Build history of the part. All positions in model axes, mm. Face numbers are marked on the shaded views. A direction names the side the tool comes from. Round coordinates to 2 decimals unless told otherwise and drop trailing zeros. Order: outer loops, then holes, each group sorted by start corner. A loop starts at its lowest first (then second) coordinate and runs counter-clockwise, first axis right, second up. Notation, with made-up numbers: M -36.75,52.5 L -17.75,52.5 A9 ccw -17.75,56.5 Z; hole C 35,-35.5 d2. An arc over 180 degrees is marked long. Use CSV: the item, a comma, the result in double quotes.
from build123d import *

# Parameters (mm, degrees)
EXTRUDE_1_DEPTH     = 10
EXTRUDE_2_DEPTH     = 10
FILLET_1_R          = 5
SKETCH_3_R          = 2.5
CUT_EXTRUDE_1_DEPTH = 10
SKETCH_4_R          = 2
CUT_EXTRUDE_2_DEPTH = 10
SKETCH_5_R          = 1.5
CUT_EXTRUDE_3_DEPTH = 10
SKETCH_6_R          = 10
CUT_EXTRUDE_4_DEPTH = 5


with BuildPart() as part:
    # 草图1 → 凸台-拉伸1 (new body)
    with BuildSketch(Plane(origin=(0, 0, 0), x_dir=(0, 0, -1), z_dir=(1, 0, 0))):
        with BuildLine():
            ThreePointArc((-7.942884534, 22.647529341), (-9.184402377, 22.17310878), (-10.397754058, 21.630689091))
            ThreePointArc((-10.397754058, 21.630689091), (-12.397305949, 24.184674774), (-15.156649968, 25.889688329))
            ThreePointArc((-15.156649968, 25.889688329), (-15.674956941, 25.579204931), (-16.186906117, 25.258346549))
            ThreePointArc((-16.186906117, 25.258346549), (-15.920443886, 22.02569307), (-14.552603542, 19.084594053))
            ThreePointArc((-14.552603542, 19.084594053), (-15.58675316, 18.249743174), (-16.573102281, 17.358925105))
            ThreePointArc((-16.573102281, 17.358925105), (-19.264014116, 19.170014316), (-22.41518439, 19.938894372))
            ThreePointArc((-22.41518439, 19.938894372), (-22.812178968, 19.48344145), (-23.199920874, 19.020085999))
            ThreePointArc((-23.199920874, 19.020085999), (-21.947555371, 16.027991201), (-19.737812321, 13.653525728))
            ThreePointArc((-19.737812321, 13.653525728), (-20.463363944, 12.539965553), (-21.126159781, 11.387948582))
            ThreePointArc((-21.126159781, 11.387948582), (-24.245026361, 12.278859291), (-27.479564388, 12.036342512))
            ThreePointArc((-27.479564388, 12.036342512), (-27.716385975, 11.480502971), (-27.941965733, 10.920006912))
            ThreePointArc((-27.941965733, 10.920006912), (-25.82628722, 8.46135788), (-22.990946508, 6.885955175))
            ThreePointArc((-22.990946508, 6.885955175), (-23.33687809, 5.602688733), (-23.611241567, 4.302240308))
            ThreePointArc((-23.611241567, 4.302240308), (-26.852766501, 4.185763967), (-29.854053162, 2.955589584))
            ThreePointArc((-29.854053162, 2.955589584), (-29.907520012, 2.353772872), (-29.948856303, 1.751001464))
            ThreePointArc((-29.948856303, 1.751001464), (-27.176962132, 0.066467896), (-23.993566664, -0.555660648))
            ThreePointArc((-23.993566664, -0.555660648), (-23.92601601, -1.883018297), (-23.785090519, -3.204601222))
            ThreePointArc((-23.785090519, -3.204601222), (-26.831970761, -4.317063099), (-29.306219208, -6.414477044))
            ThreePointArc((-29.306219208, -6.414477044), (-29.171097612, -7.003360916), (-29.024144152, -7.589404208))
            ThreePointArc((-29.024144152, -7.589404208), (-25.867366639, -8.334928429), (-22.647529341, -7.942884534))
            ThreePointArc((-22.647529341, -7.942884534), (-22.17310878, -9.184402377), (-21.630689091, -10.397754058))
            ThreePointArc((-21.630689091, -10.397754058), (-24.184674774, -12.397305949), (-25.889688329, -15.156649968))
            ThreePointArc((-25.889688329, -15.156649968), (-25.579204931, -15.674956941), (-25.258346549, -16.186906117))
            ThreePointArc((-25.258346549, -16.186906117), (-22.02569307, -15.920443886), (-19.084594053, -14.552603542))
            ThreePointArc((-19.084594053, -14.552603542), (-18.249743174, -15.58675316), (-17.358925105, -16.573102281))
            ThreePointArc((-17.358925105, -16.573102281), (-19.170014316, -19.264014116), (-19.938894372, -22.41518439))
            ThreePointArc((-19.938894372, -22.41518439), (-19.48344145, -22.812178968), (-19.020085999, -23.199920874))
            ThreePointArc((-19.020085999, -23.199920874), (-16.027991201, -21.947555371), (-13.653525728, -19.737812321))
            ThreePointArc((-13.653525728, -19.737812321), (-12.539965553, -20.463363944), (-11.387948582, -21.126159781))
            ThreePointArc((-11.387948582, -21.126159781), (-12.278859291, -24.245026361), (-12.036342512, -27.479564388))
            ThreePointArc((-12.036342512, -27.479564388), (-11.480502971, -27.716385975), (-10.920006912, -27.941965733))
            ThreePointArc((-10.920006912, -27.941965733), (-8.46135788, -25.82628722), (-6.885955175, -22.990946508))
            ThreePointArc((-6.885955175, -22.990946508), (-5.602688733, -23.33687809), (-4.302240308, -23.611241567))
            ThreePointArc((-4.302240308, -23.611241567), (-4.185763967, -26.852766501), (-2.955589584, -29.854053162))
            ThreePointArc((-2.955589584, -29.854053162), (-2.353772872, -29.907520012), (-1.751001464, -29.948856303))
            ThreePointArc((-1.751001464, -29.948856303), (-0.066467896, -27.176962132), (0.555660648, -23.993566664))
            ThreePointArc((0.555660648, -23.993566664), (1.883018297, -23.92601601), (3.204601222, -23.785090519))
            ThreePointArc((3.204601222, -23.785090519), (4.317063099, -26.831970761), (6.414477044, -29.306219208))
            ThreePointArc((6.414477044, -29.306219208), (7.003360916, -29.171097612), (7.589404208, -29.024144152))
            ThreePointArc((7.589404208, -29.024144152), (8.334928429, -25.867366639), (7.942884534, -22.647529341))
            ThreePointArc((7.942884534, -22.647529341), (9.184402377, -22.17310878), (10.397754058, -21.630689091))
            ThreePointArc((10.397754058, -21.630689091), (12.397305949, -24.184674774), (15.156649968, -25.889688329))
            ThreePointArc((15.156649968, -25.889688329), (15.674956941, -25.579204931), (16.186906117, -25.258346549))
            ThreePointArc((16.186906117, -25.258346549), (15.920443886, -22.02569307), (14.552603542, -19.084594053))
            ThreePointArc((14.552603542, -19.084594053), (15.58675316, -18.249743174), (16.573102281, -17.358925105))
            ThreePointArc((16.573102281, -17.358925105), (19.264014116, -19.170014316), (22.41518439, -19.938894372))
            ThreePointArc((22.41518439, -19.938894372), (22.812178968, -19.48344145), (23.199920874, -19.020085999))
            ThreePointArc((23.199920874, -19.020085999), (21.947555371, -16.027991201), (19.737812321, -13.653525728))
            ThreePointArc((19.737812321, -13.653525728), (20.463363944, -12.539965553), (21.126159781, -11.387948582))
            ThreePointArc((21.126159781, -11.387948582), (24.245026361, -12.278859291), (27.479564388, -12.036342512))
            ThreePointArc((27.479564388, -12.036342512), (27.716385975, -11.480502971), (27.941965733, -10.920006912))
            ThreePointArc((27.941965733, -10.920006912), (25.82628722, -8.46135788), (22.990946508, -6.885955175))
            ThreePointArc((22.990946508, -6.885955175), (23.33687809, -5.602688733), (23.611241567, -4.302240308))
            ThreePointArc((23.611241567, -4.302240308), (26.852766501, -4.185763967), (29.854053162, -2.955589584))
            ThreePointArc((29.854053162, -2.955589584), (29.907520012, -2.353772872), (29.948856303, -1.751001464))
            ThreePointArc((29.948856303, -1.751001464), (27.176962132, -0.066467896), (23.993566664, 0.555660648))
            ThreePointArc((23.993566664, 0.555660648), (23.92601601, 1.883018297), (23.785090519, 3.204601222))
            ThreePointArc((23.785090519, 3.204601222), (26.831970761, 4.317063099), (29.306219208, 6.414477044))
            ThreePointArc((29.306219208, 6.414477044), (29.171097612, 7.003360916), (29.024144152, 7.589404208))
            ThreePointArc((29.024144152, 7.589404208), (25.867366639, 8.334928429), (22.647529341, 7.942884534))
            ThreePointArc((22.647529341, 7.942884534), (22.17310878, 9.184402377), (21.630689091, 10.397754058))
            ThreePointArc((21.630689091, 10.397754058), (24.184674774, 12.397305949), (25.889688329, 15.156649968))
            ThreePointArc((25.889688329, 15.156649968), (25.579204931, 15.674956941), (25.258346549, 16.186906117))
            ThreePointArc((25.258346549, 16.186906117), (22.02569307, 15.920443886), (19.084594053, 14.552603542))
            ThreePointArc((19.084594053, 14.552603542), (18.249743174, 15.58675316), (17.358925105, 16.573102281))
            ThreePointArc((17.358925105, 16.573102281), (19.170014316, 19.264014116), (19.938894372, 22.41518439))
            ThreePointArc((19.938894372, 22.41518439), (19.48344145, 22.812178968), (19.020085999, 23.199920874))
            ThreePointArc((19.020085999, 23.199920874), (16.027991201, 21.947555371), (13.653525728, 19.737812321))
            ThreePointArc((13.653525728, 19.737812321), (12.539965553, 20.463363944), (11.387948582, 21.126159781))
            ThreePointArc((11.387948582, 21.126159781), (12.278859291, 24.245026361), (12.036342512, 27.479564388))
            ThreePointArc((12.036342512, 27.479564388), (11.480502971, 27.716385975), (10.920006912, 27.941965733))
            ThreePointArc((10.920006912, 27.941965733), (8.46135788, 25.82628722), (6.885955175, 22.990946508))
            ThreePointArc((6.885955175, 22.990946508), (5.602688733, 23.33687809), (4.302240308, 23.611241567))
            ThreePointArc((4.302240308, 23.611241567), (4.185763967, 26.852766501), (2.955589584, 29.854053162))
            ThreePointArc((2.955589584, 29.854053162), (2.353772872, 29.907520012), (1.751001464, 29.948856303))
            ThreePointArc((1.751001464, 29.948856303), (0.066467896, 27.176962132), (-0.555660648, 23.993566664))
            ThreePointArc((-0.555660648, 23.993566664), (-1.883018297, 23.92601601), (-3.204601222, 23.785090519))
            ThreePointArc((-3.204601222, 23.785090519), (-4.317063099, 26.831970761), (-6.414477044, 29.306219208))
            ThreePointArc((-6.414477044, 29.306219208), (-7.003360916, 29.171097612), (-7.589404208, 29.024144152))
            ThreePointArc((-7.589404208, 29.024144152), (-8.334928429, 25.867366639), (-7.942884534, 22.647529341))
        make_face()
    extrude(amount=EXTRUDE_1_DEPTH)

    # 草图2 → 凸台-拉伸2 (add)
    with BuildSketch(Plane(origin=(10, 0, 0), x_dir=(0, 0, -1), z_dir=(1, 0, 0))):
        Polygon((2.076731947, 90.114855515), (-4.984586669, 0.392295479), (4.984586669, -0.392295479), (12.045905284, 89.330264557), align=None)
    extrude(amount=-EXTRUDE_2_DEPTH)

    # 圆角1
    fillet_1_edges = [part.edges().sort_by_distance(p)[0] for p in [
        (5, 89.330264557, -12.045905284),
        (5, 90.114855515, -2.076731947),
    ]]
    fillet(fillet_1_edges, radius=FILLET_1_R - 0.0001)  # a hair under: the kernel refuses the full size

    # 草图3 → 切除-拉伸1 (cut)
    with BuildSketch(Plane(origin=(10, 0, 0), x_dir=(0, 0, -1), z_dir=(1, 0, 0))):
        Circle(SKETCH_3_R)
    extrude(amount=-CUT_EXTRUDE_1_DEPTH, mode=Mode.SUBTRACT)

    # 草图4 → 切除-拉伸2 (cut)
    with BuildSketch(Plane(origin=(10, 0, 0), x_dir=(0, 0, -1), z_dir=(1, 0, 0))):
        with Locations((6.669023137, 84.737973367)):
            Circle(SKETCH_4_R)
    extrude(amount=-CUT_EXTRUDE_2_DEPTH, mode=Mode.SUBTRACT)

    # 草图5 → 切除-拉伸3 (cut)
    with BuildSketch(Plane(origin=(10, 0, 0), x_dir=(0, 0, -1), z_dir=(1, 0, 0))):
        with Locations((0, 7)):
            Circle(SKETCH_5_R)
        with Locations((7, 0)):
            Circle(SKETCH_5_R)
        with Locations((0, -7)):
            Circle(SKETCH_5_R)
        with Locations((-7, 0)):
            Circle(SKETCH_5_R)
    extrude(amount=-CUT_EXTRUDE_3_DEPTH, mode=Mode.SUBTRACT)

    # 草图6 → 切除-拉伸4 (cut)
    with BuildSketch(Plane(origin=(10, 0, 0), x_dir=(0, 0, -1), z_dir=(1, 0, 0))):
        Circle(SKETCH_6_R)
    extrude(amount=-CUT_EXTRUDE_4_DEPTH, mode=Mode.SUBTRACT)


solid = part.part
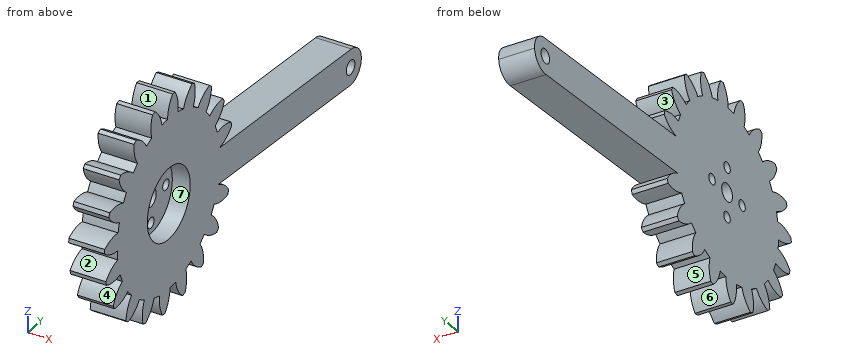
(1) Drop flat-ended pins along their axis: pin 1 (5 mm diameter, centred on x = 7.5, y = 61, fed in from +Z); pin 2 (1.5 mm diameter, centred on x = 8.5, z = 15, fed in from -Y); pin 3 (4 mm diameter, centred on x = 7, y = -7, fed in from +Z). Give the stop position or say it passes through.
Answer block:
pin 1,"stops at z = 0.41"
pin 2,"stops at y = -21.76"
pin 3,"stops at z = 29.31"
(2) Cut at A-A, the plane x = 1.75. Count the separate pieces of the cut face and the enclosed holes in it, and give its area (3 significant figures).
Answer block:
separate pieces,"1"
enclosed holes,"6"
area,"2,840 mm²"
(3) Tool access for the marked faces 4, 5, 6 and 7: list every direction of +Z, -Z, +X, -X, +Y, -Y with a clear straight run to the whole face (end or side of a thin tool).
Answer block:
face 4,"+X, -X, -Y"
face 5,"+X, -X"
face 6,"-Z, +X, -X"
face 7,"+X"
(4) Wall check: line 1 (Y direction, x = 5.5, z = 27); line 2 (Y direction, x = 1.25, z = 25); line 3 (Y direction, x = 5.25, z = 18.5). Give the ranges that are in metal, low to high. Write a range as from..to.
Answer block:
line 1,"y = -8.2..-4.42, 0..4.15, 9.61..12.15"
line 2,"y = -16.21..-13.45, -8.34..-3.5, -0.48..4.39, 7.86..12.32"
line 3,"y = -23.07..-18.02, -15.29..18.79"
(5) Cut at B-B, the plane y = 42. Give the cut face in (x, z), and give its area (3 significant figures).
Answer block:
outline,"M 0,-8.32 L 10,-8.32 L 10,1.71 L 0,1.71 Z"
area,"100 mm²"
(6) Two-plate mould, pull along Y, no slides. Class the marked faces 1, 2 and 3: released by +Y, released by -Y, zero draft, split by the parting line, or undercut.
Answer block:
face 1,"undercut"
face 2,"released by -Y"
face 3,"released by +Y"
